Could you check a few things on this drawing? It's one solid part, dimensions in mm from its lowest x, y, z. A direction names the side the tool comes from. Round coordinates to 2 decimals unless told otherwise and drop trailing zeros. Write each loop counter-clockwise with the first axis right and the second up, starting at its lowest first coordinate (ties: lowest second). Pieces come first, ordered by that corner, then holes. Notation, with made-up numbers: (-4, -15) - (8, -15) arc R23 ccw to (8, 4) - close; hole circle Ø3 at (-21.75, 26.5). An arc over 180 degrees is marked (long way). Put each result on its own line as item: value.
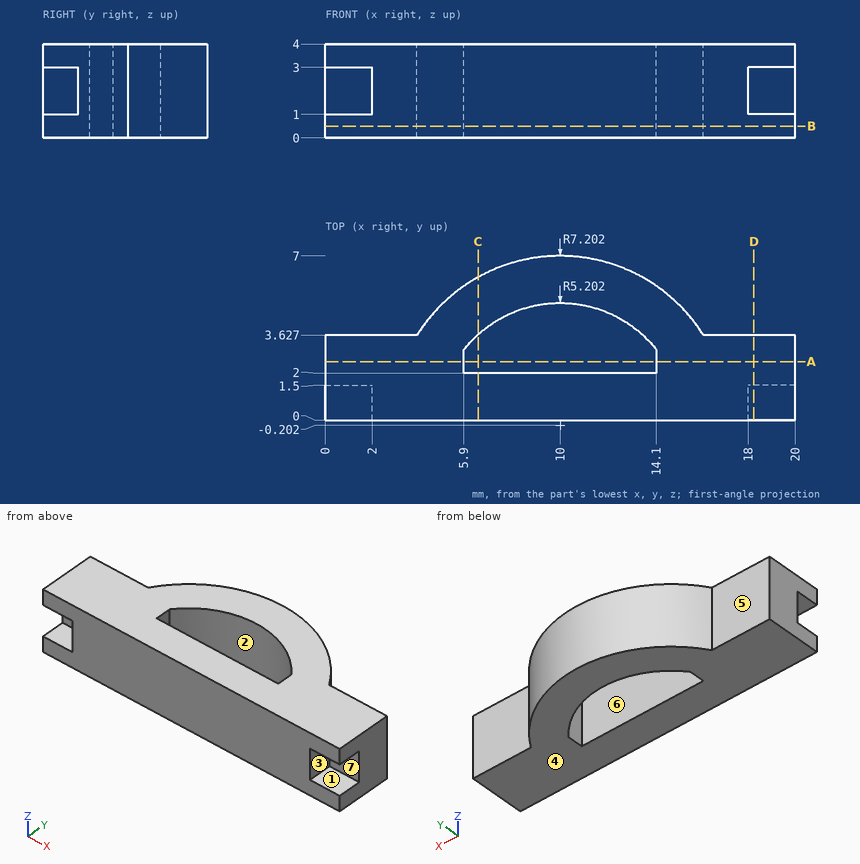
(1) Imagine slicing it at D-D, the plane x = 18.25. List the corners of the cut face in (y, z) for me, then the cut area to 3 significant figures.
Values found:
outline: (0, 0) - (3.63, 0) - (3.63, 4) - (0, 4) - (0, 3) - (1.5, 3) - (1.5, 1) - (0, 1) - close
area: 11.5 mm^2
(2) Imagine slicing it at A-A, the plane y = 2.5. List the corners of the cut face in (x, z) for me.
Values found:
outline: (0, 0) - (5.9, 0) - (5.9, 4) - (0, 4) - close; (14.1, 0) - (20, 0) - (20, 4) - (14.1, 4) - close
(3) I'm going to push flat-ended pins straight in: pin 1 (2 mm diameter, centred on y = 5.5, z = 0.5, fed in from -X) (1 decimal); pin 2 (2 mm diameter, centred on x = 17.5, z = 3, fed in from +Y); pin 3 (0.6 mm diameter, centred on x = 18.5, z = 2, fed in from -Y). Where does each tip first touch, or does it pass through?
Values found:
pin 1: stops at x = 4.5
pin 2: stops at y = 3.63
pin 3: stops at y = 1.5
(4) If we mould it in two halves opening along Z, with no side actions, what happens to the marked faces 1, 2, 3 and 4? For each: pulls with the +Z half, pulls with the -Z half, needs draft (parallel to the pull), parting line crosses it, or undercut.
Values found:
face 1: undercut
face 2: needs draft
face 3: undercut
face 4: pulls with the -Z half
(5) Imagine slicing it at C-C, the plane x = 6.5. List the corners of the cut face in (y, z) for me.
Values found:
outline: (0, 0) - (2, 0) - (2, 4) - (0, 4) - close; (3.65, 0) - (6.09, 0) - (6.09, 4) - (3.65, 4) - close
(6) Imagine slicing it at B-B, the plane z = 0.5. List the corners of the cut face in (x, y) for me (1 decimal).
Values found:
outline: (0, 0) - (20, 0) - (20, 3.6) - (16.1, 3.6) arc R7.2 ccw to (3.9, 3.6) - (0, 3.6) - close; hole (5.9, 2) - (14.1, 2) - (14.1, 3) arc R5.2 ccw to (5.9, 3) - close
(7) Please list where these lines run through material, in increasing order: probe 1 along X at (y, z) = (2.25, 2.2); probe 2 along Y at (x, z) = (17.25, 0.35); probe 3 along Y at (x, z) = (6.75, 2.8) (1 decimal). Write a range as from..to.
Values found:
probe 1: x = 0..5.9, 14.1..20
probe 2: y = 0..3.63
probe 3: y = 0..2, 3.9..6.2
(8) For the marked faces 5, 6 and 7, which set-ups out of +Z, -Z, +X, -X, +Y, -Y let a thin tool reach every point of the face, with its end or its side?
Values found:
face 5: +Z, -Z, -X, +Y
face 6: +Z, -Z
face 7: +X, -Y
